Read the model definition and answer for the solid it produces. Units are mm, in the model's axes. Coordinates: 2 decimals unless noted, no trailing zeros. Order: outer loops, then holes, each group sorted by start corner. A loop starts at its lowest first (then second) coordinate and runs counter-clockwise, first axis right, second up.
```python
from build123d import *

# Parameters (mm, degrees)
F1_R     = 1.5875
F1_R_2   = 9.525
F2_DEPTH = 12.7
F3_R     = 1.5875
F4_DEPTH = 2.54
F5_R     = 3.175


with BuildPart() as f2:
    # F1 (on Top) → F2 (new body)
    with BuildSketch(Plane.XY):
        with BuildLine():
            ThreePointArc((88.9, 273.05), (44.45, 317.5), (0, 273.05))
            Line((0, 273.05), (0, 44.45))
            ThreePointArc((0, 44.45), (44.45, 0), (88.9, 44.45))
            Line((88.9, 44.45), (88.9, 273.05))
        make_face()
        with Locations((10.853484273, 57.15)):
            Circle(F1_R, mode=Mode.SUBTRACT)
        with Locations((45.2464185655, 29.7988653183)):
            Circle(F1_R_2, mode=Mode.SUBTRACT)
        with Locations((78.2482549548, 57.15)):
            Circle(F1_R, mode=Mode.SUBTRACT)
        with Locations((10.7546523213, 224.79)):
            Circle(F1_R, mode=Mode.SUBTRACT)
        with Locations((43.8685081899, 287.5815033913)):
            Circle(F1_R_2, mode=Mode.SUBTRACT)
        with Locations((78.0730992556, 224.79)):
            Circle(F1_R, mode=Mode.SUBTRACT)
    extrude(amount=-F2_DEPTH)

    # F3 (on face) → F4 (cut)
    with BuildSketch(Plane(origin=(0, 0, -12.7), x_dir=(1, 0, 0), z_dir=(0, 0, -1))):
        with BuildLine():
            Line((0, -44.45), (0, -273.05))
            ThreePointArc((0, -273.05), (44.45, -317.5), (88.9, -273.05))
            Line((88.9, -273.05), (88.9, -44.45))
            ThreePointArc((88.9, -44.45), (44.45, 0), (0, -44.45))
        make_face()
        with Locations((10.7546523213, -224.79)):
            Circle(F3_R, mode=Mode.SUBTRACT)
        with Locations((78.0730992556, -224.79)):
            Circle(F3_R, mode=Mode.SUBTRACT)
        with BuildLine():
            Line((85.725, -241.7593711691), (85.725, -273.05))
            ThreePointArc((85.725, -273.05), (81.8143754619, -290.586506817), (70.8235307648, -304.8))
            Line((70.8235307648, -304.8), (18.0764692352, -304.8))
            ThreePointArc((18.0764692352, -304.8), (7.0856245381, -290.586506817), (3.175, -273.05))
            Line((3.175, -273.05), (3.175, -241.8057641091))
            ThreePointArc((3.175, -241.8057641091), (5.9834868143, -233.8403409002), (13.1668058106, -229.3978761248))
            Line((13.1668058106, -229.3978761248), (15.8026631116, -228.8225635949))
            ThreePointArc((15.8026631116, -228.8225635949), (19.0499999332, -224.7907424019), (15.8041137065, -220.757753291))
            Line((15.8041137065, -220.757753291), (13.1623424416, -220.1801542687))
            ThreePointArc((13.1623424416, -220.1801542687), (5.9820542559, -215.7368852391), (3.175, -207.7732413178))
            Line((3.175, -207.7732413178), (3.175, -73.9505208253))
            ThreePointArc((3.175, -73.9505208253), (6.6440839392, -65.2281250145), (15.1561320755, -61.2708824666))
            ThreePointArc((15.1561320755, -61.2708824666), (19.0324801493, -57.5298939621), (15.9075236341, -53.1417604001))
            Line((15.9075236341, -53.1417604001), (13.1716234423, -52.4694137795))
            ThreePointArc((13.1716234423, -52.4694137795), (5.6434616569, -47.1930989845), (3.648005568, -38.2191994597))
            ThreePointArc((3.648005568, -38.2191994597), (8.5202744008, -24.1354622654), (18.0764692352, -12.7))
            Line((18.0764692352, -12.7), (70.8235307648, -12.7))
            ThreePointArc((70.8235307648, -12.7), (80.4131304814, -24.1946582113), (85.2722946349, -38.3536169954))
            ThreePointArc((85.2722946349, -38.3536169954), (83.1241630177, -47.5004857983), (75.2768639326, -52.6676489864))
            Line((75.2768639326, -52.6676489864), (73.1437855148, -53.1075779034))
            ThreePointArc((73.1437855148, -53.1075779034), (69.850079032, -57.1755421779), (73.1938797929, -61.2024308286))
            Line((73.1938797929, -61.2024308286), (75.4361390988, -61.6360174279))
            ThreePointArc((75.4361390988, -61.6360174279), (82.8206997339, -66.0220738553), (85.725, -74.1050353622))
            Line((85.725, -74.1050353622), (85.725, -207.8391418625))
            ThreePointArc((85.725, -207.8391418625), (82.8133867938, -215.9309577263), (75.4135852009, -220.3124999003))
            Line((75.4135852009, -220.3124999003), (73.2012098097, -220.7361586377))
            ThreePointArc((73.2012098097, -220.7361586377), (69.8500316367, -224.7738395666), (73.1694897792, -228.8376382908))
            Line((73.1694897792, -228.8376382908), (75.5111852948, -229.3050995051))
            ThreePointArc((75.5111852948, -229.3050995051), (82.844993718, -233.7059418761), (85.725, -241.7593711691))
        make_face(mode=Mode.SUBTRACT)
        with Locations((10.853484273, -57.15)):
            Circle(F3_R, mode=Mode.SUBTRACT)
        with Locations((78.2482549548, -57.15)):
            Circle(F3_R, mode=Mode.SUBTRACT)
    extrude(amount=-F4_DEPTH, mode=Mode.SUBTRACT)

    # F5
    f5_edges = [f2.edges().sort_by_distance(p)[0] for p in [
        (35.721419, 29.798865, 0),
        (35.721419, 29.798865, -12.7),
        (34.343508, 287.581503, 0),
        (34.343508, 287.581503, -12.7),
    ]]
    fillet(f5_edges, radius=F5_R)


solid = f2.part
```
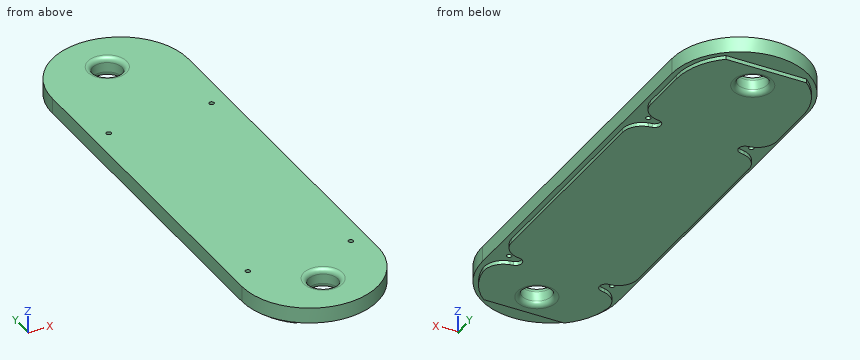
1) Straight lines are drawn through the part: line 1 (X direction, y = 224.79, z = -6); line 2 (Y direction, x = 44.5, z = -7.25); line 3 (X direction, y = 57.15, z = -6.75). For each, find the intervals that lie inside material, in ascending order.
A:
line 1: x = 0 to 9.17, 12.34 to 76.49, 79.66 to 88.9
line 2: y = 0 to 20.3, 39.29 to 278.08, 297.09 to 317.5
line 3: x = 0 to 9.27, 12.44 to 76.66, 79.84 to 88.9
2) A cutting plane is placed at A-A, the plane x = 65.5. Determine the outline of the cut face in (y, z).
A:
outline: (5.3, -10.16) - (12.7, -10.16) - (12.7, -12.7) - (304.8, -12.7) - (304.8, -10.16) - (312.2, -10.16) - (312.2, 0) - (5.3, 0) - close
3) A cutting plane is placed at B-B, the plane x = 39. State how many separate pieces and enclosed holes the cut face has, and give its area (3 significant figures).
A:
separate pieces: 3
enclosed holes: 0
area: 3,550 mm2
4) Flat-ended cylindrical pins translate along their axes: pin 1 Ø4 at (x, y) = (10.75, 224.79) entering from -Z; pin 2 Ø2 at (y, z) = (127, -12) entering from -X (3 decimals); pin 3 Ø6 at (x, z) = (79.5, -6) entering from +Y. Find the tip coordinate at first contact, or state that the pin passes through.
A:
pin 1: stops at z = -10.16
pin 2: stops at x = 3.175
pin 3: stops at y = 303.85
